Could you check a few things on this model? Use its own coordinates, in mm. A direction names the side the tool comes from. Round coordinates to 2 decimals unless told otherwise and drop trailing zeros. Loops run counter-clockwise (first coordinate to the right, second up) from the corner with the lowest first, then second, coordinate; pieces in that order, holes last. Notation, with made-up numbers: (-21, 37) - (-16, 37) arc R22 ccw to (-16, 73) - close; hole circle Ø6 at (28, -38). An arc over 180 degrees is marked (long way). Use one line per item in the form item = value.
```python
from build123d import *

# Parameters (mm, degrees)
SKETCH1_W           = 40
SKETCH1_H           = 12
BOSS_EXTRUDE1_DEPTH = 4
BOSS_EXTRUDE2_DEPTH = 12
SKETCH3_R           = 4
CUT_EXTRUDE1_DEPTH  = 13
SKETCH4_R           = 2.5
CUT_EXTRUDE2_DEPTH  = 5
FILLET1_R           = 2


with BuildPart() as part:
    # Sketch1 → Boss-Extrude1 (new body)
    with BuildSketch(Plane(origin=(0, 0, 0), x_dir=(1, 0, 0), z_dir=(0, 1, 0))):
        Rectangle(SKETCH1_W, SKETCH1_H)
    extrude(amount=BOSS_EXTRUDE1_DEPTH)

    # Sketch2 → Boss-Extrude2 (add)
    with BuildSketch(Plane.XY.offset(6)):
        with BuildLine():
            Line((20, 4), (10, 4))
            ThreePointArc((10, 4), (0, 14), (-10, 4))
            Line((-10, 4), (-20, 4))
            Line((-20, 4), (-20, 0))
            Line((-20, 0), (20, 0))
            Line((20, 0), (20, 4))
        make_face()
    extrude(amount=-BOSS_EXTRUDE2_DEPTH)

    # Sketch3 → Cut-Extrude1 (cut, through all)
    with BuildSketch(Plane.XY.offset(6)):
        with Locations((0, 7)):
            Circle(SKETCH3_R)
    extrude(amount=-CUT_EXTRUDE1_DEPTH, mode=Mode.SUBTRACT)

    # Sketch4 → Cut-Extrude2 (cut, through all)
    with BuildSketch(Plane(origin=(0, 4, 0), x_dir=(1, 0, 0), z_dir=(0, 1, 0))):
        with Locations((-15, 0)):
            Circle(SKETCH4_R)
        with Locations((15, 0)):
            Circle(SKETCH4_R)
    extrude(amount=-CUT_EXTRUDE2_DEPTH, mode=Mode.SUBTRACT)

    # Fillet1
    fillet1_edges = [part.edges().sort_by_distance(p)[0] for p in [
        (-20, 4, 0),
        (-10, 4, 0),
        (10, 4, 0),
        (20, 4, 0),
    ]]
    fillet(fillet1_edges, radius=FILLET1_R)


solid = part.part
```
1. If we section it at B-B, the plane z = 4: Write out the boundary of the cut face in (x, y), plus the area to 3 significant figures.
Solution:
outline = (-20, 0) - (20, 0) - (20, 2) arc R2 ccw to (18, 4) - (11.83, 4) arc R2 cw to (9.86, 5.67) arc R10 ccw to (-9.86, 5.67) arc R2 cw to (-11.83, 4) - (-18, 4) arc R2 ccw to (-20, 2) - close; hole circle Ø8 at (0, 7)
area = 266 mm^2
2. If we section it at D-D, the plane z = -0.5: Write out the boundary of the cut face in (x, y).
Solution:
outline = (-20, 0) - (-17.45, 0) - (-17.45, 4) - (-18, 4) arc R2 ccw to (-20, 2) - close; (-12.55, 0) - (12.55, 0) - (12.55, 4) - (11.83, 4) arc R2 cw to (9.86, 5.67) arc R10 ccw to (-9.86, 5.67) arc R2 cw to (-11.83, 4) - (-12.55, 4) - close; (17.45, 0) - (20, 0) - (20, 2) arc R2 ccw to (18, 4) - (17.45, 4) - close; hole circle Ø8 at (0, 7)
3. If we section it at C-C, the plane y = 6.25: Write out the boundary of the cut face in (x, z).
Solution:
outline = (-9.74, -6) - (-3.93, -6) - (-3.93, 6) - (-9.74, 6) - close; (3.93, -6) - (9.74, -6) - (9.74, 6) - (3.93, 6) - close
4. Please list where these lines run through material, in increasing order: line 1 along X through (y, z) = (1.65, 0); line 2 along Z through (x, y) = (-15, 2.35); line 3 along X through (y, z) = (2.9, 0).
Solution:
line_1 = -20 to -17.5, -12.5 to 12.5, 17.5 to 20
line_2 = -6 to -2.5, 2.5 to 6
line_3 = -19.79 to -17.5, -12.5 to 12.5, 17.5 to 19.79
5. For P1, Ø3, axis at y = 4, z = 0, coming from the -X side; P2, Ø5, axis at y = 6, z = 4.5, coming from the +X side; P3, Ø3, axis at x = 13, z = -2.5, coming from the +Y side, each with a flat end and sliding along its axis, tell me the tip position at first contact or that it passes through.
Solution:
P1 = -19.94
P2 = 19.32
P3 = 4.03
6. If we section it at A-A, the plane x = 15: Write out the boundary of the cut face in (y, z).
Solution:
outline = (0, -6) - (4, -6) - (4, -2.5) - (0, -2.5) - close; (0, 2.5) - (4, 2.5) - (4, 6) - (0, 6) - close
7. On a 3-axis mill with a long thin cutter (end or side, diameter ignored), from which of +Z, -Z, +X, -X, +Y, -Y can I reach the whole of each face in a straight line? I mean faces 5 (the face through (-15, 4, -3)), 6 (the face through (15, 4, 3)), 7 (the face through (12.5, 2, -0.1)). Say none if no direction works.
Solution:
face_5 = +Z, -Z, -X, +Y
face_6 = +Z, -Z, +X, +Y
face_7 = +Y, -Y
8. We'd pull the mould along Z, two halves only. Please class faces 1 (the face through (0, 2, -6)), 2 (the face through (-10.556, 4.46, -0.084)), 3 (the face through (-17.5, 2, -0.1)), 4 (the face through (0, 2, 6)): +Z half, -Z half, draft (parallel to the pull), parting line (faces both ways), or undercut.
Solution:
face_1 = -Z half
face_2 = draft
face_3 = undercut
face_4 = +Z half
